from build123d import *

# Parameters (mm, degrees)
F0_W     = 396.875
F0_H     = 304.8
F1_DEPTH = 5.55625


with BuildPart() as f1:
    # F0 (on Front) → F1 (new body)
    with BuildSketch(Plane.XZ):
        with Locations((0, 158.75)):
            Rectangle(F0_W, F0_H)
        with BuildLine():
            ThreePointArc((-50.8, 241.3), (-69.85, 260.35), (-50.8, 279.4))
            Line((-50.8, 279.4), (50.8, 279.4))
            ThreePointArc((50.8, 279.4), (64.270384, 273.820384), (69.85, 260.35))
            ThreePointArc((69.85, 260.35), (64.270384, 246.879616), (50.8, 241.3))
            Line((50.8, 241.3), (-50.8, 241.3))
        make_face(mode=Mode.SUBTRACT)
    extrude(amount=F1_DEPTH)


solid = f1.part
Geometry check sheet. Reference: the model listing, model coordinates, mm. Coordinates: 2 decimals unless noted, no trailing zeros. Order: outer loops, then holes, each group sorted by start corner. A loop starts at its lowest first (then second) coordinate and runs counter-clockwise, first axis right, second up. Notation, with made-up numbers: (-29.75, 51.5) -> (3.25, 51.5) arc R25 ccw to (3.25, 89.5) -> close; hole circle Ø7 at (-26.75, 48). An arc over 180 degrees is marked (long way). Use a Markdown table: item, result. Add a question column.
1. Mould release check, pull along X, two halves, no side actions. Record for faces 1 (the face through (-3, -5.556, 161)), 2 (the face through (-69.845, -2.739, 259.931)): pulls with the +X half, pulls with the -X half, needs draft (parallel to the pull), parting line crosses it, or undercut.
2. Material ranges on L1, parallel to Z at x = 0.5, y = -0.25; L2, parallel to Z at x = -68, y = -2.55, recorded low to high.
3. Cross-section at A-A (y = -2.55). Enter the section's corners in (x, z).
Filled sheet:
| question | item | result |
|---|---|---|
| 1 | face 1 | needs draft |
| 1 | face 2 | undercut |
| 2 | L1 | 6.35 to 241.3, 279.4 to 311.15 |
| 2 | L2 | 6.35 to 252.16, 268.54 to 311.15 |
| 3 | outline | (-198.44, 6.35) -> (198.44, 6.35) -> (198.44, 311.15) -> (-198.44, 311.15) -> close; hole (-50.8, 241.3) -> (50.8, 241.3) arc R19.05 ccw to (69.85, 260.35) arc R19.05 ccw to (50.8, 279.4) -> (-50.8, 279.4) arc R19.05 ccw to start |
